Source: three-view drawing plus pictorial views. Frame: mm from the lowest corner of the part. A direction names the side the tool comes from. Give positions to 0.01 mm unless a question says otherwise; leave off trailing zeros. Loops run counter-clockwise (first coordinate to the right, second up) from the corner with the lowest first, then second, coordinate; pieces in that order, holes last.
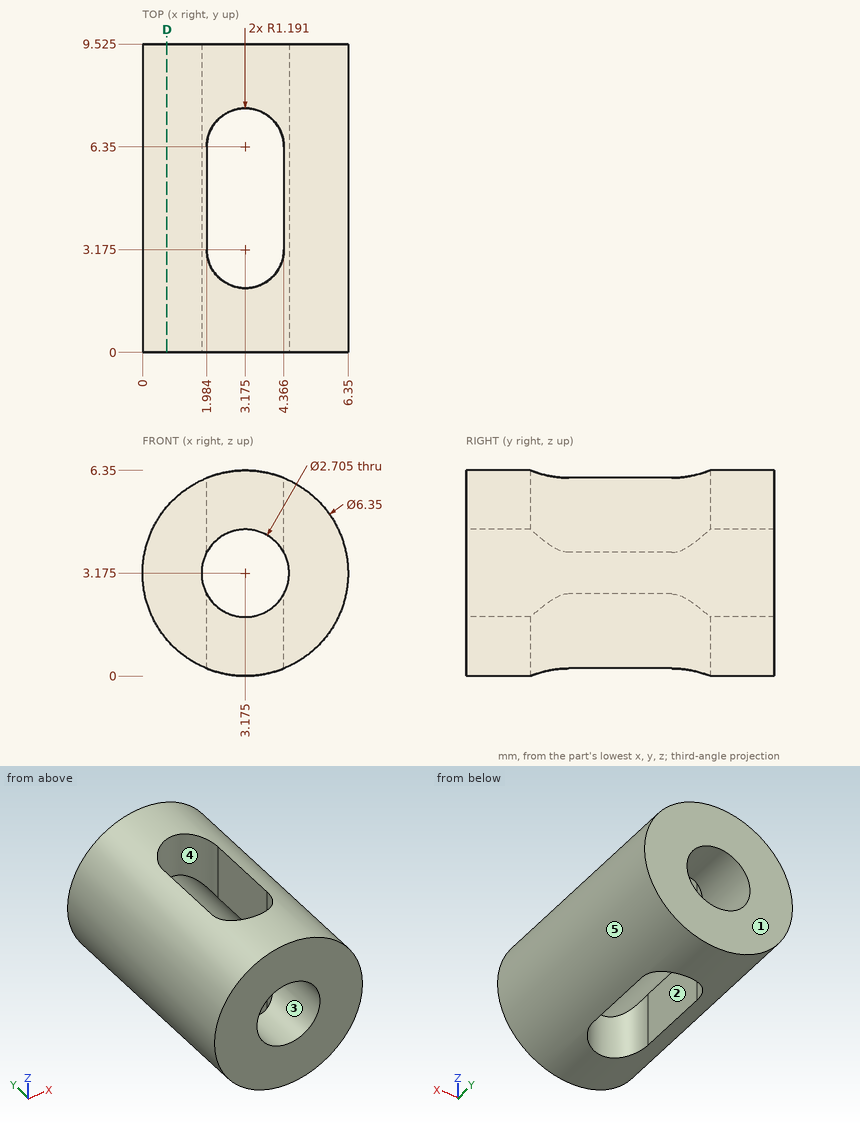
1) Reachability of the marked faces 1 and 2 from +Z, -Z, +X, -X, +Y, -Y: full face, straight path, thin tool, end or side. Return the list, or none.
Checks:
face 1: +Z, -Z, +X, -X, +Y
face 2: +Z, -Z
2) Ray query, probe 1 along X at (y, z) = (2.25, 2.5); probe 2 along X at (y, z) = (7, 1.5); probe 3 along Y at (x, z) = (4, 1.5) (1 decimal). Return the intervals inside material, ascending.
Checks:
probe 1: x = 0.07 to 2, 4.35 to 6.28
probe 2: x = 0.48 to 2.18, 4.17 to 5.87
probe 3: y = 0 to 2.3, 7.2 to 9.5
3) Cut plane D-D (x = 0.75). Return loops of the section in (y, z) (1 decimal).
Checks:
outline: (0, 1.1) - (9.5, 1.1) - (9.5, 5.2) - (0, 5.2) - close
4) Pull-direction query (Z, two-part tool) for the marked faces 3, 4 and 5; classes: released by +Z, released by -Z, zero draft, split by the parting line, or undercut.
Checks:
face 3: undercut
face 4: zero draft
face 5: split by the parting line
5) Contact query for flat-ended pins moving along their axis: P1, Ø3, axis at x = 1, y = 1.5, coming from the -Z side; P2, Ø3, axis at y = 5, z = 5.5, coming from the -X side; P3, Ø1.8, axis at y = 4, z = 1, coming from the -X side. Output: stop coordinate, or through.
Checks:
P1: stops at z = 0.07
P2: stops at x = 0.11
P3: stops at x = 0.27
